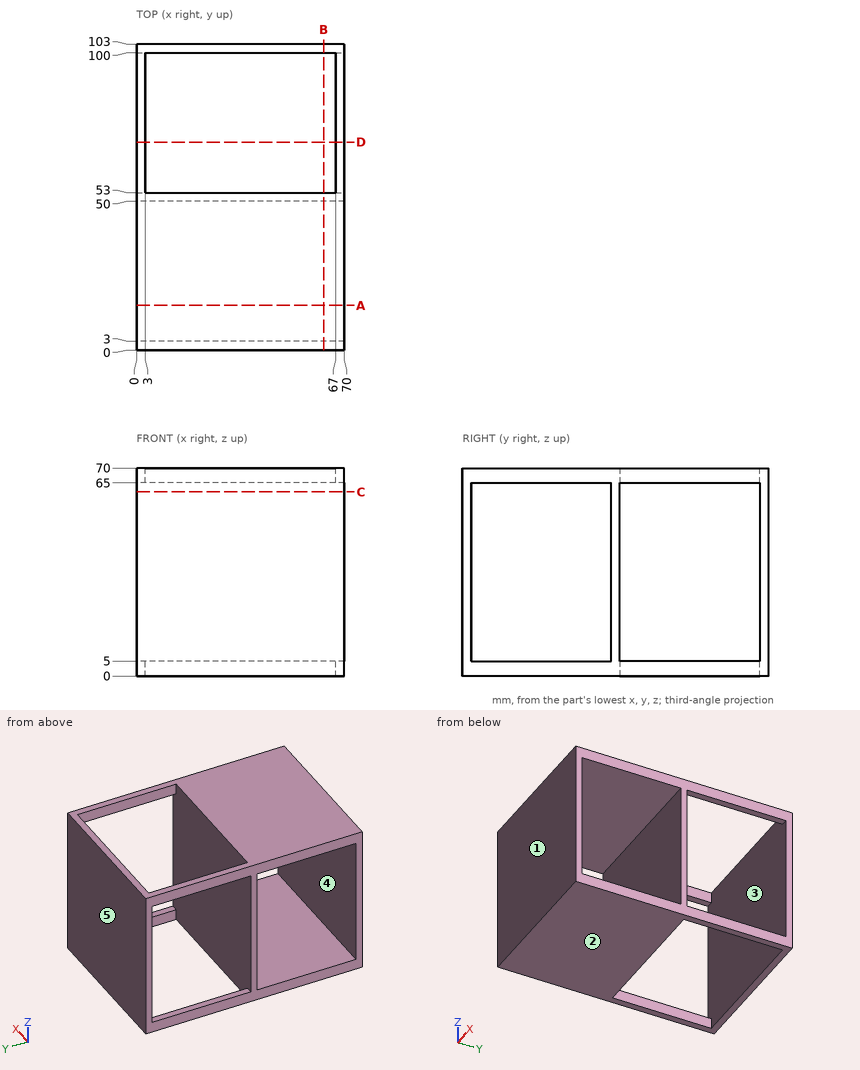
Input: dimensioned drawing with shaded views. Units: mm. Origin: part minimum x, y, z. A direction names the side the tool comes from. Coordinates: 2 decimals unless noted, no trailing zeros. Order: outer loops, then holes, each group sorted by start corner. A loop starts at its lowest first (then second) coordinate and runs counter-clockwise, first axis right, second up.
1. Cut plane A-A, the plane y = 15. Return loops of the section in (x, z), plus the area to 3 significant figures.
Checked values:
outline: (0, 0) - (70, 0) - (70, 5) - (0, 5) - close; (0, 65) - (70, 65) - (70, 70) - (0, 70) - close
area: 700 mm2
2. Ray query, line 1 along Y through (x, z) = (19, 61); line 2 along Z through (x, y) = (52.5, 48). Return the intervals inside material, ascending.
Checked values:
line 1: y = 0 to 3, 50 to 53, 100 to 103
line 2: z = 0 to 5, 65 to 70
3. Access query for the marked faces 4 and 5. Directions: +Z, -Z, +X, -X, +Y, -Y. A direction counts if a zero-diameter tool reaches every point of the face in a straight line with its end or side. Return the directions, or none.
Checked values:
face 4: +X, -X
face 5: +Z, -Z, +X, -X, +Y
4. Cut plane B-B, the plane x = 63. Return loops of the section in (y, z), plus the area to 3 significant figures.
Checked values:
outline: (0, 0) - (53, 0) - (53, 70) - (0, 70) - close; (100, 0) - (103, 0) - (103, 70) - (100, 70) - close; hole (3, 5) - (50, 5) - (50, 65) - (3, 65) - close
area: 1,100 mm2
5. Cut plane C-C, the plane z = 62. Return loops of the section in (x, y).
Checked values:
outline: (0, 0) - (70, 0) - (70, 3) - (0, 3) - close; (0, 50) - (70, 50) - (70, 53) - (0, 53) - close; (0, 100) - (70, 100) - (70, 103) - (0, 103) - close
6. Cut plane D-D, the plane y = 70. Return loops of the section in (x, z), plus the area to 3 significant figures.
Checked values:
outline: (0, 0) - (3, 0) - (3, 5) - (0, 5) - close; (0, 65) - (3, 65) - (3, 70) - (0, 70) - close; (67, 0) - (70, 0) - (70, 5) - (67, 5) - close; (67, 65) - (70, 65) - (70, 70) - (67, 70) - close
area: 60.0 mm2
7. Draft query along Y for the marked faces 1, 2 and 3. Return one class per face: +Y half, -Y half, draft (parallel to the pull), parting line (faces both ways), or undercut.
Checked values:
face 1: -Y half
face 2: draft
face 3: undercut
